Check sheet for the modelled part. Datum: model origin and axes. Units: mm. A direction names the side the tool comes from. Round coordinates to 2 decimals unless told otherwise and drop trailing zeros. Write each loop counter-clockwise with the first axis right and the second up, starting at its lowest first coordinate (ties: lowest second). Pieces come first, ordered by that corner, then holes.
Item 1: Material ranges on line 1 (X direction, y = 11.5, z = -11.5); line 2 (Y direction, x = 170, z = -10); line 3 (Z direction, x = 158.5, y = 16.75), recorded low to high.
Item 2: Cross-section at A-A on y = 21.75. Enter the section's corners in (x, z).
Item 3: Cross-section at B-B on x = 34. Enter the section's corners in (y, z).
Item 4: Release check for a two-part mould opening along X. For faces 1 (the flat face through (-31.236, 2.465, -20.774)), 2 (the flat face through (113.694, 15, -11)), 3 (the flat face through (-56.306, 2, -19)) record: +X half, -X half, draft (parallel to the pull), parting line (faces both ways), or undercut.
Item 5: Tool access check on faces 4 (the flat face through (104.694, 15, -11)), 5 (the flat face through (163.694, 15, -11)), 6 (the flat face through (159, 15, -8.379)), 7 (the flat face through (-46, 2, -8.379)), 8 (the flat face through (62, 8.75, -8)). Record the directions out of +Z, -Z, +X, -X, +Y, -Y that give a thin tool (end or side, any length) a straight path to the whole face; none if there is none.
Item 6: Go/stop test with flat-tipped pins: pin 1 Ø8 at (x, z) = (94.5, -16.5) entering from +Y; pin 2 Ø5 at (x, z) = (63, -6.5) entering from +Y; pin 3 Ø5 at (y, z) = (15.5, -13.5) entering from -X; pin 4 Ø2.5 at (x, z) = (-51.31, -13.38) entering from +Y. Record where each tip stops, or that it passes through.
from build123d import *

# Parameters (mm, degrees)
BOSS_EXTRUDE1_DEPTH = 5
SKETCH2_W           = 20
SKETCH2_H           = 10
BOSS_EXTRUDE2_DEPTH = 3.75
SKETCH3_R           = 3.775
CUT_EXTRUDE1_DEPTH  = 10
SKETCH7_R           = 1.5
CUT_EXTRUDE3_DEPTH  = 5
SKETCH4_R           = 1.5
CUT_EXTRUDE2_DEPTH  = 4
SKETCH8_W           = 9
SKETCH8_H           = 5
BOSS_EXTRUDE3_DEPTH = 20
SKETCH9_R           = 1.5
CUT_EXTRUDE4_DEPTH  = 5


with BuildPart() as part:
    # Sketch1 → Boss-Extrude1 (new body)
    with BuildSketch(Plane(origin=(0, 0, 0), x_dir=(1, 0, 0), z_dir=(0, 1, 0))):
        Polygon((-26.305830051, -6.620550836), (193.694169949, -6.620550836), (193.694169949, 13.379449164), (-26.305830051, 13.379449164), (-36.305830051, 28.379449164), (-56.305830051, 28.379449164), (-56.305830051, 8.379449164), (-36.305830051, 8.379449164), align=None)
    extrude(amount=BOSS_EXTRUDE1_DEPTH)

    # Sketch2 → Boss-Extrude2 (add)
    with BuildSketch(Plane(origin=(0, 5, 0), x_dir=(1, 0, 0), z_dir=(0, 1, 0))):
        with Locations((68.694169949, 8.379449164)):
            Rectangle(SKETCH2_W, SKETCH2_H)
    extrude(amount=BOSS_EXTRUDE2_DEPTH)

    # Sketch3 → Cut-Extrude1 (cut)
    with BuildSketch(Plane.XY.offset(-3.379449164)):
        with Locations((68.694169949, 8.75)):
            Circle(SKETCH3_R)
    extrude(amount=-CUT_EXTRUDE1_DEPTH, mode=Mode.SUBTRACT)

    # Sketch7 → Cut-Extrude3 (cut)
    with BuildSketch(Plane(origin=(0, 5, 0), x_dir=(1, 0, 0), z_dir=(0, 1, 0))):
        with Locations(Location((-51.305830051, 23.379449164, 0), (0, 0, 270))):
            Circle(SKETCH7_R)
        with Locations(Location((-51.305830051, 13.379449164, 0), (0, 0, 270))):
            Circle(SKETCH7_R)
        with Locations(Location((188.694169949, -1.620550836, 0), (0, 0, 270))):
            Circle(SKETCH7_R)
        with Locations(Location((188.694169949, 8.379449164, 0), (0, 0, 270))):
            Circle(SKETCH7_R)
        with Locations(Location((183.694169949, 3.379449164, 0), (0, 0, 270))):
            Circle(SKETCH7_R)
        with Locations(Location((-46.305830051, 18.379449164, 0), (0, 0, 270))):
            Circle(SKETCH7_R)
    extrude(amount=-CUT_EXTRUDE3_DEPTH, mode=Mode.SUBTRACT)

    # Sketch4 → Cut-Extrude2 (cut)
    with BuildSketch(Plane(origin=(0, 8.75, 0), x_dir=(1, 0, 0), z_dir=(0, 1, 0))):
        with Locations(Location((75.694169949, 6.379449164, 0), (0, 0, 270))):
            Circle(SKETCH4_R)
        with Locations(Location((61.694169949, 10.379449164, 0), (0, 0, 270))):
            Circle(SKETCH4_R)
    extrude(amount=-CUT_EXTRUDE2_DEPTH, mode=Mode.SUBTRACT)

    # Sketch8 → Boss-Extrude3 (add)
    with BuildSketch(Plane(origin=(0, 5, 0), x_dir=(1, 0, 0), z_dir=(0, 1, 0))):
        with Locations((109.194169949, 10.879449164)):
            Rectangle(SKETCH8_W, SKETCH8_H)
        with Locations((159.194169949, 10.879449164)):
            Rectangle(SKETCH8_W, SKETCH8_H)
    extrude(amount=BOSS_EXTRUDE3_DEPTH)

    # Sketch9 → Cut-Extrude4 (cut)
    with BuildSketch(Plane.XY.offset(-8.379449164)):
        with Locations((108.894169949, 17.5)):
            Circle(SKETCH9_R)
        with Locations((159.494169949, 8)):
            Circle(SKETCH9_R)
    extrude(amount=-CUT_EXTRUDE4_DEPTH, mode=Mode.SUBTRACT)


solid = part.part
Response values:
1. line 1: x = 104.69 to 113.69, 154.69 to 163.69
1. line 2: y = 0 to 5
1. line 3: z = -13.38 to -8.38
2. outline: (104.69, -13.38) - (113.69, -13.38) - (113.69, -8.38) - (104.69, -8.38) - close; (154.69, -13.38) - (163.69, -13.38) - (163.69, -8.38) - (154.69, -8.38) - close
3. outline: (0, -13.38) - (5, -13.38) - (5, 6.62) - (0, 6.62) - close
4. face 1: +X half
4. face 2: undercut
4. face 3: -X half
5. face 4: +Z, -Z, +Y
5. face 5: +Z, -Z, +X, +Y
5. face 6: +Z, +X, +Y
5. face 7: +Z, -X, +Y, -Y
5. face 8: +Z, -Z, -X, +Y
6. pin 1: stops at y = 5
6. pin 2: stops at y = 8.75
6. pin 3: stops at x = 104.69
6. pin 4: passes through
